Here's how the part is built. I have some questions about the finished solid (model axes, mm). Face numbers are marked on the shaded views. A direction names the side the tool comes from. Round coordinates to 2 decimals unless told otherwise and drop trailing zeros. Order: outer loops, then holes, each group sorted by start corner. A loop starts at its lowest first (then second) coordinate and runs counter-clockwise, first axis right, second up. Notation, with made-up numbers: M 6,-21 L 37,-21 A27 cw 37,18 Z; hole C 7,-15.5 d7. An arc over 180 degrees is marked long. Write item = value, one per line. Start each with the question number.
Item 1: Please list where these lines run through material, in increasing order: L1, parallel to X at y = 2.5, z = 0; L2, parallel to Z at x = 0, y = 8.45.
Item 2: We'd pull the mould along Y, two halves only. Please class the marked faces 3, 4, 5 and 6: pulls with the +Y half, pulls with the -Y half, needs draft (parallel to the pull), parting line crosses it, or undercut.
Item 3: For the marked faces 1 and 2, which set-ups out of +Z, -Z, +X, -X, +Y, -Y let a thin tool reach every point of the face, with its end or its side?
Item 4: I want a section at A-A, the plane x = 0. List the corners of the cut face in (y, z) for me.
Item 5: I'm going to push flat-ended pins straight in: P1, Ø8, axis at x = -7.5, z = 7.5, coming from the -Y side; P2, Ø3, axis at x = 6, y = 8.5, coming from the +Z side; P3, Ø5, axis at y = 8, z = 4.5, coming from the -X side; P4, Ø1.5, axis at x = 2, z = 2.5, coming from the -Y side. Where does each tip first touch, or does it pass through?
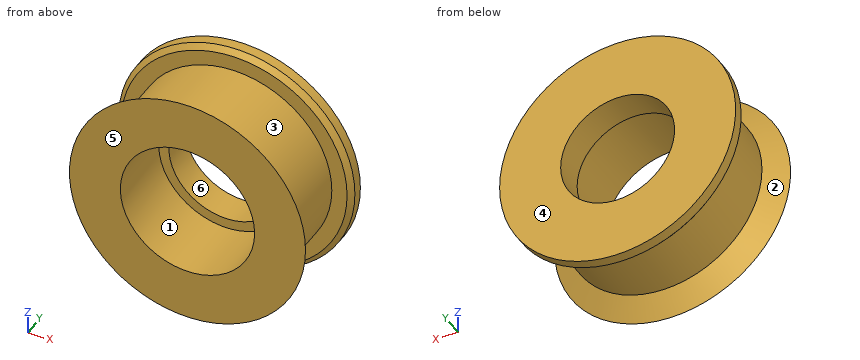
Autodesk Inventor part; units mm, degrees
ref_plane "YZ Plane" through (0, 0, 0) normal (1, 0, 0) x (0, 1, 0)
ref_plane "XZ Plane" through (0, 0, 0) normal (0, 1, 0) x (-1, 0, 0)
ref_plane "XY Plane" through (0, 0, 0) normal (0, 0, 1) x (1, 0, 0)
sketch "Sketch1" plane through (0, 0, 0) normal (0, 0, 1) x (1, 0, 0)
  line L0 (6.6, 0) -> (11.6, 0)
  line L1 (11.6, 0) -> (11.6, 10) construction
  line L2 (11.6, 10) -> (6.6, 10)
  line L3 (6.6, 10) -> (6.6, 0)
  line L4 (0, 0) -> (0, 8.5122) construction
  line L5 (9.6, 8.5) -> (9.6, 1.5)
  line L6 (9.6, 8.5) -> (11.1, 8.5)
  line L7 (11.1, 8.5) -> (11.6, 9)
  line L8 (11.6, 0) -> (9.6, 1.5)
  line L9 (11.6, 9) -> (11.6, 10)
  line L10 (6.6, 10) -> (5.6, 10)
  line L11 (5.6, 10) -> (5.6, 7)
  line L12 (5.6, 7) -> (6.6, 7)
  line L13 (6.6, 7) -> (6.6, 10)
  point P0 (11.6, 0.6699)
  point P1 (11.6, 5)
  point P2 (15.2143, 7.5754)
  point P3 (15.2143, 2.4246)
  point P4 (9.6, 5)
  point P5 (17.7886, 0.302)
  point P6 (6.6, 5)
  dimension "d6" = 10
  dimension "d7" = 6.6
  dimension "d14" = 5
  dimension "d17" = 7
  dimension "d18" = 1.5
  dimension "d19" = 135
  dimension "d20" = 2
  dimension "d21" = 1
  dimension "d22" = 3
revolve "Revolution1" add sketch "Sketch1" angle 360 about axis through (0, 0, 0) along (0, 1, 0)
properties part number "pully10mmx20mmx12mm"
Filled in:
q1.L1 = -9.6 to -6.6, 6.6 to 9.6
q1.L2 = -9.6 to -5.6, 5.6 to 9.6
q2.face_3 = undercut
q2.face_4 = pulls with the +Y half
q2.face_5 = pulls with the -Y half
q2.face_6 = needs draft
q3.face_1 = -Y
q3.face_2 = none
q4.outline = M 0,-11.6 L 1.5,-9.6 L 8.5,-9.6 L 8.5,-11.1 L 9,-11.6 L 10,-11.6 L 10,-5.6 L 7,-5.6 L 7,-6.6 L 0,-6.6 Z; M 0,6.6 L 7,6.6 L 7,5.6 L 10,5.6 L 10,11.6 L 9,11.6 L 8.5,11.1 L 8.5,9.6 L 1.5,9.6 L 0,11.6 Z
q5.P1 = 0
q5.P2 = 10.66
q5.P3 = -11.39
q5.P4 = through
